```python
from build123d import *

# Parameters (mm, degrees)
CUT_EXTRUDE1_DEPTH = 2
FILLET1_R          = 0.5


with BuildPart() as part:
    # Sketch2 → Revolve1 (revolve)
    with BuildSketch(Plane.XY):
        Polygon((0, 0), (2.65, 0), (2.65, 3), (1.4, 3), (1.4, 33), (0, 33), align=None)
    revolve(axis=Axis((0, 0, 0), (0, 1, 0)))

    # Sketch3 → Cut-Extrude1 (cut)
    with BuildSketch(Plane.XZ):
        Polygon((-1.443375673, 0), (-0.721687836, -1.25), (0.721687836, -1.25), (1.443375673, 0), (0.721687836, 1.25), (-0.721687836, 1.25), align=None)
    extrude(amount=-CUT_EXTRUDE1_DEPTH, mode=Mode.SUBTRACT)

    # Sketch4 → Cut-Revolve1 (revolve, cut)
    with BuildSketch(Plane(origin=(0, 0, 0), x_dir=(-1, 0, 0), z_dir=(0, 0, -1))):
        with BuildLine():
            Line((0, 0), (0, 0.3))
            ThreePointArc((0, 0.3), (-0.887764045, 0.22445693), (-1.75, 0))
            Line((-1.75, 0), (0, 0))
        make_face()
    revolve(axis=Axis((0, 0, 0), (0, 1, 0)), mode=Mode.SUBTRACT)

    # Fillet1
    fillet1_edges = [part.edges().sort_by_distance(p)[0] for p in [
        (-2.65, 0, 0),
    ]]
    fillet(fillet1_edges, radius=FILLET1_R)


solid = part.part
```
Check sheet for the modelled part. Datum: model origin and axes. Units: mm. A direction names the side the tool comes from. Round coordinates to 2 decimals unless told otherwise and drop trailing zeros. Loops run counter-clockwise (first coordinate to the right, second up) from the corner with the lowest first, then second, coordinate; pieces in that order, holes last. Notation, with made-up numbers: (24, 54) - (77, 54) arc R14 ccw to (77, 66) - close; hole circle Ø1 at (3.5, 53). An arc over 180 degrees is marked (long way). Answer as a JSON object with one key per item and string values. Group by question number.
Q1. Scan lines: line 1 along Y through (x, z) = (0.5, 1.2); line 2 along Z through (x, y) = (1.2, 14.5); line 3 along Z through (x, y) = (-0.05, 28). Record each from-to range of solid material in increasing order. Write a range as [from, to].
Q2. Gauge pin test, flat ends, axial feed: P1, Ø1.5, axis at x = 2, z = -1, coming from the +Y side; P2, Ø1, axis at x = 1, y = 23.5, coming from the +Z side. Record the tip position at first contact, or that the pin passes through.
Q3. Sectioned sample at B-B, the plane y = 24.5. Enter the section's corners in (x, z).
Q4. Set-up check for faces 4 (the face through (0, 1, -1.25)), 5 (the face through (0, 33, 0)): record each of +Z, -Z, +X, -X, +Y, -Y from which the full face is reachable in a straight line by a thin tool's end or side.
Q5. Sectioned sample at A-A, the plane x = 0. Enter the section's corners in (y, z), plus the area to 3 significant figures.
Q6. Mould release check, pull along Z, two halves, no side actions. Record for faces 1 (the face through (-1.4, 18.21, -0.06)), 2 (the face through (1.1, 3, 1.1)), 3 (the face through (1.088, 1.036, 0.616)): released by +Z, released by -Z, zero draft, split by the parting line, or undercut.
Solution:
{
 "1": {"line 1": "y = [2, 33]", "line 2": "z = [-0.72, 0.72]", "line 3": "z = [-1.4, 1.4]"},
 "2": {"P1": "stops at y = 3", "P2": "stops at z = 1.31"},
 "3": {"outline": "circle Ø2.8 at (0, 0)"},
 "4": {"face 4": "-Y", "face 5": "+Z, -Z, +X, -X, +Y"},
 "5": {"outline": "(0, -2.15) arc R0.5 ccw to (0.5, -2.65) - (3, -2.65) - (3, -1.4) - (33, -1.4) - (33, 1.4) - (3, 1.4) - (3, 2.65) - (0.5, 2.65) arc R0.5 ccw to (0, 2.15) - (0, 1.75) arc R5.25 cw to (0.15, 1.25) - (2, 1.25) - (2, -1.25) - (0.15, -1.25) arc R5.25 cw to (0, -1.75) - close", "area": "94.7 mm²"},
 "6": {"face 1": "split by the parting line", "face 2": "zero draft", "face 3": "undercut"}
}
